Could you check a few things on this model? Use its own coordinates, in mm. Round coordinates to 2 decimals unless told otherwise and drop trailing zeros. Order: outer loops, then holes, each group sorted by start corner. A loop starts at its lowest first (then second) coordinate and runs counter-clockwise, first axis right, second up. Notation, with made-up numbers: (71.25, 31.25) -> (127.25, 31.25) arc R21 ccw to (127.25, 43.25) -> close; hole circle Ø6 at (-11.75, 16.25). An arc over 180 degrees is marked (long way). One line per question, with ' | ' between items.
Autodesk Inventor part; units mm, degrees
ref_plane "YZ Plane" through (0, 0, 0) normal (1, 0, 0) x (0, 1, 0)
ref_plane "XZ Plane" through (0, 0, 0) normal (0, 1, 0) x (-1, 0, 0)
ref_plane "XY Plane" through (0, 0, 0) normal (0, 0, 1) x (1, 0, 0)
sketch "スケッチ1" plane through (0, 0, 0) normal (0, 1, 0) x (-1, 0, 0)
  line L0 (0, 0) -> (84, 0)
  line L1 (84, 0) -> (84, 230)
  line L2 (84, 230) -> (0, 230)
  line L3 (0, 230) -> (0, 0)
  dimension "d0" = 84
  dimension "d1" = 230
extrude "押し出し1" add sketch "スケッチ1" along normal blind 2
sketch "スケッチ2" plane through (0, 2, 0) normal (0, 1, 0) x (1, 0, 0)
  line L0 (0, 0) -> (-84, 0)
  line L1 (0, -230) -> (0, 0)
  circle A0 centre (-42, -224) radius 2.65
  line L2 (-84, -230) -> (0, -230)
  circle A1 centre (-42, -176) radius 2.65
  circle A2 centre (-28.5, -2) radius 1.1
  circle A3 centre (-28.5, -20.5) radius 1.1
  circle A4 centre (-55.5, -15.5) radius 1.1
  circle A5 centre (-42, -200) radius 10
  dimension "d9" = 5.3
  dimension "d10" = 6
  dimension "d11" = 42
  dimension "d12" = 5.3
  dimension "d13" = 48
  dimension "d16" = 2.2
  dimension "d17" = 2.2
  dimension "d18" = 2.2
  dimension "d19" = 228
  dimension "d20" = 209.5
  dimension "d21" = 214.5
  dimension "d22" = 55.5
  dimension "d23" = 28.5
  dimension "d24" = 28.5
  dimension "d27" = 20
  dimension "d28" = 24
extrude "押し出し5" cut sketch "スケッチ2" against normal blind 2
properties part number "Force_Arm_board"
1. I need wall thicknesses on probe 1 along Z at (x, y) = (-42, 0.75); probe 2 along Z at (x, y) = (-28.5, 1.05); probe 3 along X at (y, z) = (0.9, 20.5). Which ranges of each line are inside material? Lowest first, please.
From the geometry:
probe 1: z = 0 to 173.35, 178.65 to 190, 210 to 221.35, 226.65 to 230 | probe 2: z = 0 to 0.9, 3.1 to 19.4, 21.6 to 230 | probe 3: x = -84 to -29.6, -27.4 to 0
2. I want a section at A-A on z = 176. List the corners of the cut face in (x, y) for me.
From the geometry:
outline: (-84, 0) -> (-44.65, 0) -> (-44.65, 2) -> (-84, 2) -> close; (-39.35, 0) -> (0, 0) -> (0, 2) -> (-39.35, 2) -> close
3. I want a section at C-C on z = 200. List the corners of the cut face in (x, y) for me, and give its area (3 significant figures).
From the geometry:
outline: (-84, 0) -> (-52, 0) -> (-52, 2) -> (-84, 2) -> close; (-32, 0) -> (0, 0) -> (0, 2) -> (-32, 2) -> close | area: 128 mm²
4. If we mould it in two halves opening along X, with no side actions, what happens to faces 1 (the face through (-41, 0, 117)), 2 (the face through (-42.34, 1.01, 221.37))? For each: pulls with the +X half, pulls with the -X half, needs draft (parallel to the pull), parting line crosses it, or undercut.
From the geometry:
face 1: needs draft | face 2: undercut
5. I want a section at B-B on y = 1.7. List the corners of the cut face in (x, z) for me.
From the geometry:
outline: (-84, 0) -> (0, 0) -> (0, 230) -> (-84, 230) -> close; hole circle Ø2.2 at (-55.5, 15.5); hole circle Ø20 at (-42, 200); hole circle Ø5.3 at (-42, 176); hole circle Ø5.3 at (-42, 224); hole circle Ø2.2 at (-28.5, 2); hole circle Ø2.2 at (-28.5, 20.5)
6. I'm going to push a flat-ended pin straight in: pin 1 (5 mm diameter, centred on x = -29, z = 173.5, fed in from -Y). Where does the tip first touch, or does it pass through?
From the geometry:
pin 1: stops at y = 0
